from build123d import *

# Parameters (mm, degrees)
SKETCH1_W           = 55
SKETCH1_H           = 65
BOSS_EXTRUDE1_DEPTH = 27.5
SHELL1_T            = -2
SKETCH2_W           = 51
SKETCH2_H           = 61
CUT_EXTRUDE1_DEPTH  = 68.981615162


with BuildPart() as part:
    # Sketch1 → Boss-Extrude1 (new, symmetric)
    with BuildSketch(Plane.XY):
        Rectangle(SKETCH1_W, SKETCH1_H)
    extrude(amount=BOSS_EXTRUDE1_DEPTH, both=True)

    # Shell1
    shell1_openings = [part.faces().sort_by_distance(p)[0] for p in [
        (0, 0, 27.5),
    ]]
    offset(amount=SHELL1_T, openings=shell1_openings, kind=Kind.INTERSECTION)

    # Sketch2 → Cut-Extrude1 (cut, through all)
    with BuildSketch(Plane.XY.offset(-25.5)):
        Rectangle(SKETCH2_W, SKETCH2_H)
    extrude(amount=-CUT_EXTRUDE1_DEPTH, mode=Mode.SUBTRACT)


solid = part.part
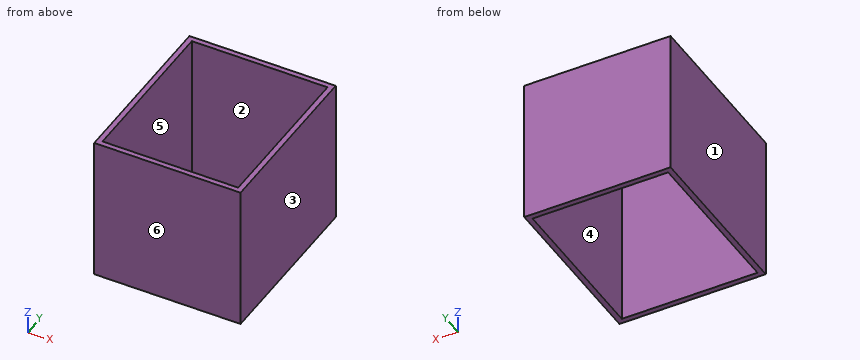
Verification items for the finished model (mm, model axes). Face numbers are marked on the shaded views. A direction names the side the tool comes from. Coordinates: 2 decimals unless noted, no trailing zeros. Order: outer loops, then holes, each group sorted by start corner. A loop starts at its lowest first (then second) coordinate and runs counter-clockwise, first axis right, second up. Notation, with made-up numbers: M -38.75,-21 L -10.75,-21 A20 ccw -10.75,13 Z; hole C 12.25,4.5 d5. An arc over 180 degrees is marked long. One line per item, written item: value. Start each with the question number.
Item 1: Sectioned sample at B-B on x = -20.5. Record the cut outline in (y, z), then the cut area to 3 significant figures.
Item 2: Sectioned sample at A-A on y = -4. Record the cut outline in (x, z), then the cut area to 3 significant figures.
Item 3: Access from +Z, -Z, +X, -X, +Y, -Y to the whole of each face (thin tool, end or side, straight path). Record for the marked faces 1 and 2.
Item 4: Mould release check, pull along X, two halves, no side actions. Record for the marked faces 3, 4, 5 and 6: pulls with the +X half, pulls with the -X half, needs draft (parallel to the pull), parting line crosses it, or undercut.
Item 5: Thickness scan on probe 1 along X at (y, z) = (29, -3); probe 2 along Y at (x, z) = (17, -24). Record the ranges inside material, lowest first.
Item 6: Sectioned sample at C-C on z = -18. Record the cut outline in (x, y), then the cut area to 3 significant figures.
Calculated:
1. outline: M -32.5,-27.5 L -30.5,-27.5 L -30.5,27.5 L -32.5,27.5 Z; M 30.5,-27.5 L 32.5,-27.5 L 32.5,27.5 L 30.5,27.5 Z
1. area: 220 mm^2
2. outline: M -27.5,-27.5 L -25.5,-27.5 L -25.5,27.5 L -27.5,27.5 Z; M 25.5,-27.5 L 27.5,-27.5 L 27.5,27.5 L 25.5,27.5 Z
2. area: 220 mm^2
3. face 1: +Z, -Z, -X, +Y, -Y
3. face 2: +Z, -Z
4. face 3: pulls with the +X half
4. face 4: undercut
4. face 5: undercut
4. face 6: needs draft
5. probe 1: -27.5 to -25.5, 25.5 to 27.5
5. probe 2: -32.5 to -30.5, 30.5 to 32.5
6. outline: M -27.5,-32.5 L 27.5,-32.5 L 27.5,32.5 L -27.5,32.5 Z; hole M -25.5,-30.5 L 25.5,-30.5 L 25.5,30.5 L -25.5,30.5 Z
6. area: 464 mm^2
